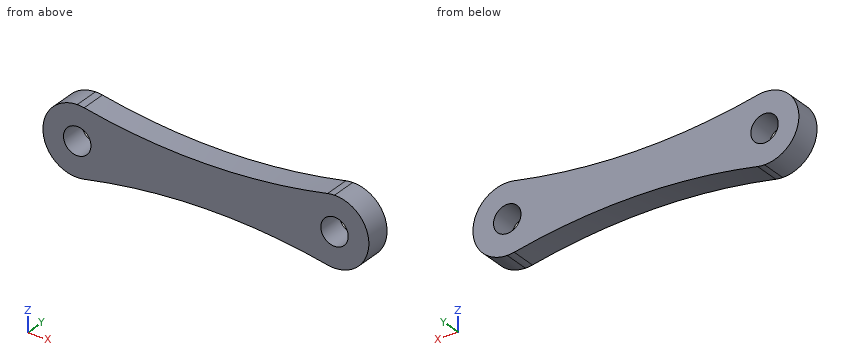
```python
from build123d import *
from build123d.topology import SkipClean

# Parameters (mm, degrees)
SKETCH1_R           = 0.8
BOSS_EXTRUDE1_DEPTH = 1.5
SKETCH2_OUTSIDE_W   = 24.894
SKETCH2_OUTSIDE_H   = 9.894
CUT_EXTRUDE1_DEPTH  = 10.823441352


with BuildPart() as part:
    # Sketch1 → Boss-Extrude1 (new body)
    with BuildSketch(Plane(origin=(0, 0, 0), x_dir=(1, 0, 0), z_dir=(0, 1, 0))):
        with BuildLine():
            Line((-7.5, 2), (7.5, 2))
            ThreePointArc((7.5, 2), (9.5, 0), (7.5, -2))
            Line((7.5, -2), (-7.5, -2))
            ThreePointArc((-7.5, -2), (-9.5, 0), (-7.5, 2))
        make_face()
        with Locations(Location((-7.5, 0, 0), (0, 0, 270))):
            Circle(SKETCH1_R, mode=Mode.SUBTRACT)
        with Locations(Location((7.5, 0, 0), (0, 0, 270))):
            Circle(SKETCH1_R, mode=Mode.SUBTRACT)
    extrude(amount=BOSS_EXTRUDE1_DEPTH)

    # Sketch2 outside → Cut-Extrude1 (cut, through all)
    with SkipClean():  # the faces are left unmerged after this step: merging them gives an invalid solid
        with BuildSketch(Plane(origin=(0, 1.5, 0), x_dir=(1, 0, 0), z_dir=(0, 1, 0))):
            Rectangle(SKETCH2_OUTSIDE_W, SKETCH2_OUTSIDE_H)
            with BuildLine():
                ThreePointArc((-7.094594595, 1.95848065), (-9.5, 0), (-7.094594595, -1.95848065))
                ThreePointArc((-7.094594595, -1.95848065), (0, -1.231892029), (7.094594595, -1.95848065))
                ThreePointArc((7.094594595, -1.95848065), (9.5, 0), (7.094594595, 1.95848065))
                ThreePointArc((7.094594595, 1.95848065), (0, 1.231892029), (-7.094594595, 1.95848065))
            make_face(mode=Mode.SUBTRACT)
        extrude(amount=-CUT_EXTRUDE1_DEPTH, mode=Mode.SUBTRACT)


solid = part.part
```
Could you check a few things on this model? Use its own coordinates, in mm. Round coordinates to 2 decimals unless told otherwise and drop trailing zeros. Loops run counter-clockwise (first coordinate to the right, second up) from the corner with the lowest first, then second, coordinate; pieces in that order, holes last. Notation, with made-up numbers: (3, -5) - (39, -5) arc R9 cw to (39, 1) - close; hole circle Ø6 at (65.5, 64.25). An arc over 180 degrees is marked (long way). Answer in a Markdown table with one row per item. Add a question column.
(1) I need wall thicknesses on line 1 along X through (y, z) = (1.15, 0); line 2 along X through (y, z) = (0.25, 0.5); line 3 along Z through (x, y) = (0, 0.8). Which ranges of each line are inside material? Lowest first, please.
(2) If we section it at B-B (y = 0.8): Please give me the cut outline in (x, z).
(3) I'm going to push a flat-ended pin straight in: pin 1 (2 mm diameter, centred on x = -7.5, z = 0, fed in from -Y). Where does the tip first touch, or does it pass through?
(4) If we section it at D-D (z = -1): Please give me the cut outline in (x, y), plus the area to 3 significant figures.
(5) If we section it at A-A (z = 0): Please give me the cut outline in (x, y).
(6) If we section it at C-C (z = 1.55): Please give me the cut outline in (x, y).
Model answer:
| question | item | result |
|---|---|---|
| 1 | line 1 | x = -9.5 to -8.3, -6.7 to 6.7, 8.3 to 9.5 |
| 1 | line 2 | x = -9.44 to -8.12, -6.88 to 6.88, 8.12 to 9.44 |
| 1 | line 3 | z = -1.23 to 1.23 |
| 2 | outline | (-7.09, -1.96) arc R35 cw to (7.09, -1.96) arc R2 ccw (long way) to (7.09, 1.96) arc R35 cw to (-7.09, 1.96) arc R2 ccw (long way) to start; hole circle Ø1.6 at (-7.5, 0); hole circle Ø1.6 at (7.5, 0) |
| 3 | pin 1 | stops at y = 0 |
| 4 | outline | (-9.23, 0) - (9.23, 0) - (9.23, 1.5) - (-9.23, 1.5) - close |
| 4 | area | 27.7 mm² |
| 5 | outline | (-9.5, 0) - (-8.3, 0) - (-8.3, 1.5) - (-9.5, 1.5) - close; (-6.7, 0) - (6.7, 0) - (6.7, 1.5) - (-6.7, 1.5) - close; (8.3, 0) - (9.5, 0) - (9.5, 1.5) - (8.3, 1.5) - close |
| 6 | outline | (-8.76, 0) - (-4.71, 0) - (-4.71, 1.5) - (-8.76, 1.5) - close; (4.71, 0) - (8.76, 0) - (8.76, 1.5) - (4.71, 1.5) - close |
